from build123d import *

# Parameters (mm, degrees)
F1_DEPTH = 70
F3_DEPTH = 25
F4_R     = 1
F5_R     = 1
F6_W     = 24.6687295064
F6_H     = 11.3869960284
F7_DEPTH = 5


with BuildPart() as f1:
    # F0 (on Top) → F1 (new body)
    with BuildSketch(Plane.XY):
        Polygon((0, 25), (0, 0), (25, 0), (25, 1.5), (1.5, 1.5), (1.5, 25), align=None)
    extrude(amount=F1_DEPTH)

    # F2 (on Front) → F3 (join)
    with BuildSketch(Plane.XZ):
        Polygon((0, 25), (0, 0), (25, 0), (25, 1.5), (1.5, 1.5), (1.5, 25), align=None)
    extrude(amount=-F3_DEPTH)

    # F4
    f4_edges = [f1.edges().sort_by_distance(p)[0] for p in [
        (0, 0, 35),
        (0, 12.5, 0),
        (12.5, 0, 0),
    ]]
    fillet(f4_edges, radius=F4_R)

    # F5
    f5_edges = [f1.edges().sort_by_distance(p)[0] for p in [
        (25, 13, 0),
        (13, 25, 0),
        (25, 25, 0.75),
    ]]
    fillet(f5_edges, radius=F5_R)

    # F6 (on face) → F7 (cut)
    with BuildSketch(Plane(origin=(0, 0, 0), x_dir=(1, 0, 0), z_dir=(0, 0, -1))):
        with Locations((29.8343647532, -23.1934980142)):
            Rectangle(F6_W, F6_H)
    extrude(amount=-F7_DEPTH, mode=Mode.SUBTRACT)


solid = f1.part
Source: CAD feature listing. Evaluate the final solid. Frame: model axes, mm. A direction names the side the tool comes from. Give positions to 0.01 mm unless a question says otherwise; leave off trailing zeros. Order: outer loops, then holes, each group sorted by start corner. A loop starts at its lowest first (then second) coordinate and runs counter-clockwise, first axis right, second up. Notation, with made-up numbers: (85, 44.25) -> (142, 44.25) arc R31 ccw to (142, 71.25) -> close; hole circle Ø2 at (76.5, 85.5). An arc over 180 degrees is marked (long way). Write item = value, one per line.
Q1. Cut plane A-A, the plane y = 4. Output: boundary loops of the cut face in (x, z).
Data:
outline = (0, 1) arc R1 ccw to (1, 0) -> (24, 0) arc R1 ccw to (25, 1) -> (25, 1.5) -> (1.5, 1.5) -> (1.5, 70) -> (0, 70) -> close
Q2. Pin query (flat end, axial travel): pin 1 (1.2 mm diameter, centred on x = 22, z = 1, fed in from +Y); pin 2 (0.8 mm diameter, centred on y = 22, z = 0.5, fed in from +X); pin 3 (8 mm diameter, centred on x = 8.5, y = 22, fed in from +Z). Return the tip coordinate at first contact, or that it passes through.
Data:
pin_1 = 17.5
pin_2 = 17.5
pin_3 = 1.5
Q3. Cut plane B-B, the plane z = 33.5. Output: boundary loops of the cut face in (x, y), and give its area (3 significant figures).
Data:
outline = (0, 1) arc R1 ccw to (1, 0) -> (24, 0) arc R1 ccw to (25, 1) -> (25, 1.5) -> (1.5, 1.5) -> (1.5, 25) -> (1, 25) arc R1 ccw to (0, 24) -> close
area = 72.1 mm^2
Q4. Set-up query: faces 1 (the face through (13, 13, 1.5)), 2 (the face through (12, 0, 35)), 3 (the face through (17.5, 21, 1)). Return all of +Z, -Z, +X, -X, +Y, -Y with unobstructed straight access to the full face (end or side cutting, diameter ignored); none if empty.
Data:
face_1 = +Z, +X, +Y
face_2 = +Z, -Z, +X, -X, -Y
face_3 = +Z, -Z, +X, +Y
Q5. Cut plane D-D, the plane x = 18.25. Output: boundary loops of the cut face in (y, z).
Data:
outline = (0, 1) arc R1 ccw to (1, 0) -> (17.5, 0) -> (17.5, 1.5) -> (1.5, 1.5) -> (1.5, 70) -> (0, 70) -> close
Q6. Material intervals for line 1 (Y direction, x = 7.75, z = 23.5), sorted ascending. Write a range as from..to.
Data:
line_1 = 0..1.5
